```python
from build123d import *

# Parameters (mm, degrees)
SKETCH4_R                    = 25.6
BOSS_EXTRUDE5_DEPTH          = 2.6
SKETCH5_R                    = 16.25
BOSS_EXTRUDE6_DEPTH          = 1.2
SKETCH6_R                    = 12.25
BOSS_EXTRUDE7_DEPTH          = 8.8
SKETCH7_R                    = 7.5
BOSS_EXTRUDE8_DEPTH          = 3
FILLET2_R                    = 0.5
CUT_EXTRUDE1_DEPTH           = 0.8
CHAMFER2_SIZE                = 0.8
M2_5_CLEARANCE_HOLE1_D       = 2.9
CIRPATTERN1_COUNT            = 3
CHAMFER2_OF_CIRPATTERN1_SIZE = 0.8
CIRPATTERN2_COUNT            = 6
SKETCH13_R                   = 18.75
BOSS_EXTRUDE9_DEPTH          = 2
SKETCH14_R                   = 17.75
BOSS_EXTRUDE10_DEPTH         = 5
CUT_EXTRUDE3_START           = -1.8
CUT_EXTRUDE3_DEPTH           = 1.8
FILLET6_R                    = 2
FILLET8_R                    = 1


# Some blends are built 0.0001 mm under size
with BuildPart() as part:
    # Sketch4 → Boss-Extrude5 (new body)
    with BuildSketch(Plane.XY):
        Circle(SKETCH4_R)
    extrude(amount=BOSS_EXTRUDE5_DEPTH)

    # Sketch5 → Boss-Extrude6 (add)
    with BuildSketch(Plane.XY.offset(2.6)):
        Circle(SKETCH5_R)
    extrude(amount=BOSS_EXTRUDE6_DEPTH)

    # Sketch6 → Boss-Extrude7 (add)
    with BuildSketch(Plane.XY.offset(3.8)):
        Circle(SKETCH6_R)
    extrude(amount=BOSS_EXTRUDE7_DEPTH)

    # Sketch7 → Boss-Extrude8 (add)
    with BuildSketch(Plane.XY.offset(12.6)):
        Circle(SKETCH7_R)
    extrude(amount=BOSS_EXTRUDE8_DEPTH)

    # Fillet2
    fillet2_edges = [part.edges().sort_by_distance(p)[0] for p in [
        (-25.6, 0, 0),
    ]]
    fillet(fillet2_edges, radius=FILLET2_R)

    # Sketch8 → Cut-Extrude1 (cut)
    with BuildSketch(Plane.XY.offset(2.6)):
        with BuildLine():
            Line((3.9, -23.210366581), (3.9, -30.789633419))
            ThreePointArc((3.9, -30.789633419), (0, -34.689633419), (-3.9, -30.789633419))
            Line((-3.9, -30.789633419), (-3.9, -23.210366581))
            ThreePointArc((-3.9, -23.210366581), (0, -19.310366581), (3.9, -23.210366581))
        make_face()
    cut_extrude1 = extrude(amount=-CUT_EXTRUDE1_DEPTH, mode=Mode.SUBTRACT)

    # Chamfer2
    chamfer2_edges = [part.edges().sort_by_distance(p)[0] for p in [
        (-3.9, -24.255776162, 2.6),
        (0, -19.310366581, 2.6),
        (3.9, -24.255776162, 2.6),
    ]]
    chamfer(chamfer2_edges, length=CHAMFER2_SIZE - 0.0001)  # a hair under: the kernel refuses the full size

    # M2.5 Clearance Hole1 (through all)
    with Locations(Plane.XY.offset(1.8)):
        with Locations((0, -23)):
            m2_5_clearance_hole1 = Hole(M2_5_CLEARANCE_HOLE1_D / 2)

    # CirPattern1: Cut-Extrude1, M2.5 Clearance Hole1 ×3 about axis
    cirpattern1_axis = Axis((0, 0, 0), (0, 0, 1))
    add([cut_extrude1.rotate(cirpattern1_axis, i * 360 / CIRPATTERN1_COUNT) for i in range(1, CIRPATTERN1_COUNT)], mode=Mode.SUBTRACT)
    add([m2_5_clearance_hole1.rotate(cirpattern1_axis, i * 360 / CIRPATTERN1_COUNT) for i in range(1, CIRPATTERN1_COUNT)], mode=Mode.SUBTRACT)

    # Chamfer2 of CirPattern1
    chamfer2_of_cirpattern1_edges = [part.edges().sort_by_distance(p)[0] for p in [
        (22.956118345, 8.750389006, 2.6),
        (16.723268015, 9.65518329, 2.6),
        (19.056118345, 15.505387156, 2.6),
        (-19.056118345, 15.505387156, 2.6),
        (-16.723268015, 9.65518329, 2.6),
        (-22.956118345, 8.750389006, 2.6),
    ]]
    chamfer(chamfer2_of_cirpattern1_edges, length=CHAMFER2_OF_CIRPATTERN1_SIZE - 0.0001)  # a hair under: the kernel refuses the full size

    # Sketch12 → Tap Drill for M2x0.4 Tap1 (revolve, cut)
    with BuildSketch(Plane(origin=(0, -10.25, 12.6), x_dir=(0, -1, 0), z_dir=(1, 0, 0))):
        Polygon((0, 0), (0, 6.480688495), (0.8, 6), (0.8, 0), align=None)
    tap_drill_for_m2x0_4_tap1 = revolve(axis=Axis((0, -10.25, 18.95), (0, 0, -1)), mode=Mode.SUBTRACT)

    # CirPattern2: Tap Drill for M2x0.4 Tap1 ×6 about axis
    cirpattern2_axis = Axis((0, 0, 0), (0, 0, 1))
    for i in range(1, CIRPATTERN2_COUNT):
        add(tap_drill_for_m2x0_4_tap1.rotate(cirpattern2_axis, i * 360 / CIRPATTERN2_COUNT), mode=Mode.SUBTRACT)

    # Sketch13 → Boss-Extrude9 (add)
    with BuildSketch(Plane(origin=(0, 0, 0), x_dir=(-1, 0, 0), z_dir=(0, 0, -1))):
        with Locations(Location((0, 0, 0), (0, 0, 180))):
            Circle(SKETCH13_R)
    extrude(amount=BOSS_EXTRUDE9_DEPTH)

    # Sketch14 → Boss-Extrude10 (add)
    with BuildSketch(Plane(origin=(0, 0, -2), x_dir=(-1, 0, 0), z_dir=(0, 0, -1))):
        Circle(SKETCH14_R)
    extrude(amount=BOSS_EXTRUDE10_DEPTH)

    # Sketch17 → Cut-Extrude3 (cut)
    with BuildSketch(Plane(origin=(0, 0, -7), x_dir=(-1, 0, 0), z_dir=(0, 0, -1)).offset(CUT_EXTRUDE3_START)):
        with BuildLine():
            Line((-0.28156747, -7.28156747), (-2.121320344, -9.121320344))
            ThreePointArc((-2.121320344, -9.121320344), (-2.707106781, -10.535533906), (-2.121320344, -11.949747468))
            Line((-2.121320344, -11.949747468), (3.358335088, -17.4294029))
            ThreePointArc((3.358335088, -17.4294029), (12.551145366, -12.551145366), (17.4294029, -3.358335088))
            Line((17.4294029, -3.358335088), (11.949747468, 2.121320344))
            ThreePointArc((11.949747468, 2.121320344), (10.535533906, 2.707106781), (9.121320344, 2.121320344))
            Line((9.121320344, 2.121320344), (7.28156747, 0.28156747))
            ThreePointArc((7.28156747, 0.28156747), (7.075303297, -0.018410953), (6.99008997, -0.372346897))
            ThreePointArc((6.99008997, -0.372346897), (4.949747468, -4.949747468), (0.372346897, -6.99008997))
            ThreePointArc((0.372346897, -6.99008997), (0.018410953, -7.075303297), (-0.28156747, -7.28156747))
        make_face()
    extrude(amount=CUT_EXTRUDE3_DEPTH, mode=Mode.SUBTRACT)

    # Fillet6
    # the kernel refuses this fillet: 2 mm, written as the material it takes off along each edge
    with BuildSketch(Plane(origin=(-17.4294029, -3.358335088, -5.2), x_dir=(-0.05717413002562378, 0.9983642215423252, 0), z_dir=(0, 0, -1))) as fillet6_piece_1:
        with BuildLine():
            CenterArc((4.447159251, 1.982298833), FILLET6_R, 138.277623698, 139.350968751)
            Line((2.954402599, 3.313342625), (0, 0))
            ThreePointArc((0, 0), (2.356330648, -0.157097855), (4.712661296, 0))
        make_face()
    extrude(amount=13.58165324, mode=Mode.SUBTRACT)
    with BuildSketch(Plane(origin=(-3.358335088, -17.4294029, -5.2), x_dir=(0.9983642215423252, -0.057174130025623736, 0), z_dir=(0, 0, -1))) as fillet6_piece_2:
        with BuildLine():
            CenterArc((4.447159251, -1.982298833), FILLET6_R, 82.371407551, 139.350968751)
            Line((2.954402599, -3.313342625), (0, 0))
            ThreePointArc((0, 0), (2.356330648, 0.157097855), (4.712661296, 0))
        make_face()
    extrude(amount=13.58165324, mode=Mode.SUBTRACT)

    # Fillet8
    fillet8_edges = [part.edges().sort_by_distance(p)[0] for p in [
        (-10.535533906, 2.707106781, -7),
        (-8.201443907, 1.201443907, -7),
        (-7.075303297, -0.018410953, -7),
        (-4.949747468, -4.949747468, -7),
        (-0.018410953, -7.075303297, -7),
        (1.201443907, -8.201443907, -7),
        (2.707106781, -10.535533906, -7),
        (0.950996294, -13.120071518, -7),
        (-13.120071518, 0.950996294, -7),
        (12.551145366, 12.551145366, -7),
        (-0.622487974, -16.539565739, -7),
        (-16.539565739, -0.622487974, -7),
    ]]
    fillet(fillet8_edges, radius=FILLET8_R)


solid = part.part
```
The listing builds one solid part. Answer for the finished solid, in the listing's coordinates (mm). A direction names the side the tool comes from. Round coordinates to 2 decimals unless told otherwise and drop trailing zeros. Write each loop counter-clockwise with the first axis right and the second up, starting at its lowest first coordinate (ties: lowest second). Pieces come first, ordered by that corner, then holes. Notation, with made-up numbers: (30, -31) -> (82, -31) arc R8 cw to (82, -17) -> close; hole circle Ø2 at (-14, 19). An arc over 180 degrees is marked (long way). Write item = value, one per line.
1) For a pull along Y with two mould halves and no side action, classify faces 5 (the flat face through (5, 6, 12.6)), 6 (the cylindrical face through (-20.3, -15.6, 1.5)), 7 (the conical face through (-8.82, 5, 6.2)) as released by +Y, released by -Y, zero draft, split by the parting line, or undercut.
Check values:
face_5 = zero draft
face_6 = split by the parting line
face_7 = undercut
2) Section A-A on z = -4 is taken. Write down the section's boundary in (x, y), plus the area to 3 significant figures.
Check values:
outline = circle Ø35.5 at (0, 0)
area = 990 mm²
3) Section B-B on z = 14 is taken. Write down the section's boundary in (x, y), plus the area to 3 significant figures.
Check values:
outline = circle Ø15 at (0, 0)
area = 177 mm²
4) Given pin 1 (1.9 mm diameter, centred on x = 0, y = -21, fed in from +Z); pin 2 (2 mm diameter, centred on x = 8.88, y = 5.12, fed in from +Z); pin 3 (2.5 mm diameter, centred on x = -8.88, y = -5.13, fed in from -Z), each flat-ended and moving along its own axis, determine where each tip first touches the part or whether it passes through.
Check values:
pin_1 = 1.8
pin_2 = 12.6
pin_3 = -5.2
5) Straight lines are drawn through the part: line 1 along Z through (x, y) = (-4, -17.5); line 2 along Z through (x, y) = (3.5, 11); line 3 along X through (y, z) = (-10.25, 9.4). For each, find the intervals that lie inside material, in ascending order. Write a range as [from, to].
Check values:
line_1 = [-2, 2.6]
line_2 = [-7, 12.6]
line_3 = [-6.71, -0.8], [0.8, 6.71]
6) Which of the six approach directions +Z, -Z, +X, -X, +Y, -Y give full straight-line access (tool end or side, diameter ignored) to faces 1 (the cylindrical face through (-8.2, -4.7, 9.6)), 2 (the flat face through (-18.87, 15.85, 2.19)), 3 (the flat face through (4, 4, -7)), 4 (the cylindrical face through (1.147, -13.349, -6.715))?
Check values:
face_1 = +Z
face_2 = +Z, -X
face_3 = -Z, +X, -X, +Y, -Y
face_4 = -Z, -X
